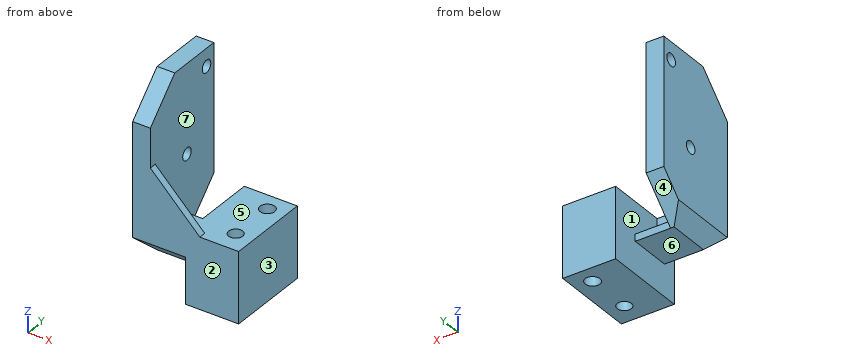
from build123d import *

# Parameters (mm, degrees)
EXTRUDE_1_DEPTH     = 12
CUT_EXTRUDE_1_REACH = 22
SKETCH_2_R          = 2
SKETCH_3_W          = 46
SKETCH_3_H          = 26
SKETCH_3_R          = 1.75
EXTRUDE_2_DEPTH     = 5
CHAMFER_1_SIZE      = 10
EXTRUDE_3_DEPTH     = 2
CHAMFER_2_SIZE      = 10
SKETCH_5_W          = 15
SKETCH_5_H          = 20
EXTRUDE_4_DEPTH     = 12
SKETCH_6_R          = 2.084127943
CUT_EXTRUDE_2_DEPTH = 21
SKETCH_7_W          = 10
SKETCH_7_H          = 5
CUT_EXTRUDE_3_DEPTH = 47
SKETCH_8_W          = 10
SKETCH_8_H          = 9
EXTRUDE_5_DEPTH     = 2
CHAMFER_3_SIZE      = 4


with BuildPart() as part:
    # Эскиз1 → Бобышка-Вытянуть1 (new body)
    with BuildSketch(Plane(origin=(0, 0, 0), x_dir=(1, 0, 0), z_dir=(0, 1, 0))):
        Polygon((0, 0), (0, 11), (15, 11), (15, 20), (30, 20), (30, 0), align=None)
    extrude(amount=EXTRUDE_1_DEPTH)

    # Эскиз2 → Вырез-Вытянуть1 (cut, up to next)
    with BuildSketch(Plane.XY, mode=Mode.PRIVATE) as cut_extrude_1_sk1:
        with Locations((25, 6)):
            Circle(SKETCH_2_R)
    cut_extrude_1_tool1 = extrude(cut_extrude_1_sk1.sketch, amount=-CUT_EXTRUDE_1_REACH, mode=Mode.PRIVATE) & part.part
    add(cut_extrude_1_tool1.solids().sort_by_distance((25, 6, 0))[0], mode=Mode.SUBTRACT)

    # Эскиз3 → Бобышка-Вытянуть2 (add)
    with BuildSketch(Plane.ZY):
        with Locations((12, 13)):
            Rectangle(SKETCH_3_W, SKETCH_3_H)
        with Locations((30, 23)):
            Circle(SKETCH_3_R, mode=Mode.SUBTRACT)
        with Locations((10, 15)):
            Circle(SKETCH_3_R, mode=Mode.SUBTRACT)
    extrude(amount=-EXTRUDE_2_DEPTH)

    # Фаска1
    chamfer_1_edges = [part.edges().sort_by_distance(p)[0] for p in [
        (2.5, 26, -11),
    ]]
    chamfer(chamfer_1_edges, length=CHAMFER_1_SIZE)

    # Эскиз4 → Бобышка-Вытянуть3 (add)
    with BuildSketch(Plane.XZ):
        Polygon((5, 14), (19, 0), (5, 0), align=None)
    extrude(amount=-EXTRUDE_3_DEPTH)

    # Фаска2
    chamfer_2_edges = [part.edges().sort_by_distance(p)[0] for p in [
        (2.5, 0, 35),
    ]]
    chamfer(chamfer_2_edges, length=CHAMFER_2_SIZE)

    # Эскиз5 → Бобышка-Вытянуть4 (add)
    with BuildSketch(Plane(origin=(0, 12, 0), x_dir=(1, 0, 0), z_dir=(0, 1, 0))):
        with Locations((22.5, 10)):
            Rectangle(SKETCH_5_W, SKETCH_5_H)
    extrude(amount=EXTRUDE_4_DEPTH)

    # Эскиз6 → Вырез-Вытянуть2 (cut, through all)
    with BuildSketch(Plane.XY):
        with Locations((25, 19)):
            Circle(SKETCH_6_R)
    extrude(amount=-CUT_EXTRUDE_2_DEPTH, mode=Mode.SUBTRACT)

    # Эскиз7 → Вырез-Вытянуть3 (cut, through all)
    with BuildSketch(Plane(origin=(0, 0, -11), x_dir=(-1, 0, 0), z_dir=(0, 0, -1))):
        with Locations((-10, 9.5)):
            Rectangle(SKETCH_7_W, SKETCH_7_H)
    extrude(amount=-CUT_EXTRUDE_3_DEPTH, mode=Mode.SUBTRACT)

    # Эскиз8 → Бобышка-Вытянуть5 (add)
    with BuildSketch(Plane(origin=(0, 0, -11), x_dir=(-1, 0, 0), z_dir=(0, 0, -1))):
        with Locations((-10, 11.5)):
            Rectangle(SKETCH_8_W, SKETCH_8_H)
    extrude(amount=-EXTRUDE_5_DEPTH)

    # Фаска3
    chamfer_3_edges = [part.edges().sort_by_distance(p)[0] for p in [
        (0, 8, -11),
        (7.5, 0, -11),
    ]]
    chamfer(chamfer_3_edges, length=CHAMFER_3_SIZE)


solid = part.part
For this review, take the finished solid that the model builds, in its own axes (mm). Face numbers are marked on the shaded views. A direction names the side the tool comes from. Round coordinates to 2 decimals unless told otherwise and drop trailing zeros. Order: outer loops, then holes, each group sorted by start corner. A loop starts at its lowest first (then second) coordinate and runs counter-clockwise, first axis right, second up. Notation, with made-up numbers: M -19,52.25 L 15,52.25 A27 cw 15,79.25 Z; hole C -24,-27.5 d1. An arc over 180 degrees is marked long. Use a Markdown table: item, result. Add a question column.
Item 1: Mouldability with a two-part tool opening along X and no side actions: class the marked faces 1, 2 and 3 as released by +X, released by -X, zero draft, split by the parting line, or undercut.
Item 2: Add section A-A, the plane y = 6. Give the boundary of the cut face in (x, z), then the cut area to 3 significant figures.
Item 3: Add section C-C, the plane x = 25. Give the boundary of the cut face in (y, z).
Item 4: Insertion check: pin 1 (4.5 mm diameter, centred on y = 15, z = 10, fed in from +X); pin 2 (7 mm diameter, centred on x = 11.5, y = 6.5, fed in from +Z); pin 3 (9 mm diameter, centred on x = 7, y = 10, fed in from -Z). Each pin has a flat end and moves straight along its axis. Give the tip position at first contact, or say it passes through.
Item 5: To check wall thickness, follow line 1 along Y through (x, z) = (3.35, 30); line 2 along Y through (x, z) = (25, -6.25); line 3 along X through (y, z) = (8.75, -4). State the ranges of each line that lie inside material, in increasing order.
Item 6: Add section B-B, the plane z = 30. Give the boundary of the cut face in (x, y).
Item 7: Add section D-D, the plane y = 23. Give the boundary of the cut face in (x, z).
Item 8: Tool access review of the marked faces 4, 5, 6 and 7: name each direction out of +Z, -Z, +X, -X, +Y, -Y from which nothing blocks a thin tool from reaching the whole face with its end or side.
Geometry results:
| question | item | result |
|---|---|---|
| 1 | face 1 | undercut |
| 1 | face 2 | zero draft |
| 1 | face 3 | released by +X |
| 2 | outline | M 0,-7 L 4,-11 L 15,-11 L 15,-20 L 23,-20 L 23,0 L 5,0 L 5,31 L 0,31 Z; M 27,-20 L 30,-20 L 30,0 L 27,0 Z |
| 2 | area | 532 mm² |
| 3 | outline | M 0,-20 L 4,-20 L 4,0 L 0,0 Z; M 8,-20 L 16.92,-20 L 16.92,0 L 8,0 Z; M 21.08,-20 L 24,-20 L 24,0 L 21.08,0 Z |
| 4 | pin 1 | stops at x = 5 |
| 4 | pin 2 | stops at z = 0 |
| 4 | pin 3 | stops at z = -11 |
| 5 | line 1 | y = 5 to 21.25, 24.75 to 26 |
| 5 | line 2 | y = 0 to 4, 8 to 16.92, 21.08 to 24 |
| 5 | line 3 | x = 0 to 5, 15 to 30 |
| 6 | outline | M 0,5 L 5,5 L 5,21.25 L 0,21.25 Z; M 0,24.75 L 5,24.75 L 5,26 L 0,26 Z |
| 7 | outline | M 0,-4 L 5,-4 L 5,28.25 L 0,28.25 Z; M 0,31.75 L 5,31.75 L 5,35 L 0,35 Z; M 15,-20 L 30,-20 L 30,0 L 15,0 Z |
| 8 | face 4 | -Z, -X, +Y |
| 8 | face 5 | +Z, +X, +Y |
| 8 | face 6 | -Z, -X, +Y, -Y |
| 8 | face 7 | +Z, +Y |
